Input: part model. Units: mm. Frame: model coordinates. Face numbers are marked on the shaded views. Round coordinates to 2 decimals unless told otherwise and drop trailing zeros. Loops run counter-clockwise (first coordinate to the right, second up) from the corner with the lowest first, then second, coordinate; pieces in that order, holes last.
1) Section B-B, the plane z = 0. Return loops of the section in (x, y).
2) Section C-C, the plane y = -35. Return loops of the section in (x, z).
3) First-contact query: pin 1 (1.5 mm diameter, centred on x = -31.5, y = -41.5, fed in from -Z). Flat tip, straight axial feed; report the tip coordinate or a pass-through.
4) Section A-A, the plane x = 0. Return loops of the section in (y, z), and give its area (3 significant figures).
5) Ray query, line 1 along Z through (x, y) = (0, -13); line 2 along Z through (x, y) = (3.5, -42.5); line 3 along X through (y, z) = (-47.5, -14). Return the intervals inside material, ascending.
6) Section D-D, the plane x = -30. Return loops of the section in (y, z), and give its area (3 significant figures).
7) Draft query along X for the marked faces 1, 2 and 3. Return one class per face: pulls with the +X half, pulls with the -X half, needs draft (parallel to the pull), parting line crosses it, or undercut.
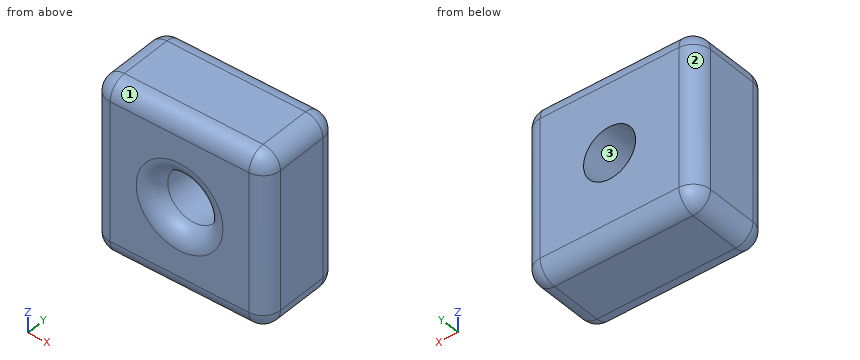
from build123d import *

# Parameters (mm, degrees)
F0_W     = 100
F0_H     = 100
F0_R     = 15
F1_DEPTH = 50
F2_R     = 10
F3_DEPTH = 50
F6_R     = 10


# Not quite as in the source:
# - the program builds the solid bodies; features that only make, move or delete a surface that nothing else refers to are left out


with BuildPart() as f1:
    # F0 (on Front) → F1 (new body, symmetric)
    with BuildSketch(Plane.XZ):
        Rectangle(F0_W, F0_H)
        Circle(F0_R, mode=Mode.SUBTRACT)
    extrude(amount=F1_DEPTH, both=True)

    # F2
    f2_edges = [f1.edges().sort_by_distance(p)[0] for p in [
        (50, 50, 0),
        (50, 0, 50),
        (50, -50, 0),
        (50, 0, -50),
        (0, -50, 50),
        (-50, -50, 0),
        (0, -50, -50),
        (-15, -50, 0),
        (0, 50, 50),
        (-50, 0, 50),
        (-50, 50, 0),
        (-50, 0, -50),
    ]]
    fillet(f2_edges, radius=F2_R)

    # F0 (on Front) → F3 (cut)
    with BuildSketch(Plane.XZ):
        Rectangle(F0_W, F0_H)
        Circle(F0_R, mode=Mode.SUBTRACT)
    extrude(amount=-F3_DEPTH, mode=Mode.SUBTRACT)

    # F6
    f6_edges = [f1.edges().sort_by_distance(p)[0] for p in [
        (-47.071068, 0, -47.071068),
        (-40, -20, -50),
        (-47.071068, -40, -47.071068),
        (-50, -20, -40),
        (-47.071068, 0, 47.071068),
        (-40, -20, 50),
        (-47.071068, -40, 47.071068),
        (-50, -20, 40),
        (-47.071068, -47.071068, 40),
        (-50, -40, 0),
        (-40, -50, 0),
        (-47.071068, -47.071068, -40),
        (-50, 0, 0),
        (47.071068, -40, -47.071068),
        (50, -20, -40),
        (47.071068, 0, -47.071068),
        (40, -20, -50),
        (50, -40, 0),
        (50, -20, 40),
        (50, 0, 0),
        (40, -50, 0),
        (0, -50, -40),
        (0, -50, 40),
        (-25, -50, 0),
        (0, 0, 50),
        (47.071068, 0, 47.071068),
        (0, 0, -50),
    ]]
    fillet(f6_edges, radius=F6_R)


solid = f1.part
Final values:
1. outline: (-50, -40) arc R10 ccw to (-40, -50) - (-25, -50) arc R10 ccw to (-15, -40) - (-15, 0) - (-40, 0) arc R10 ccw to (-50, -10) - close; (15, -40) arc R10 ccw to (25, -50) - (40, -50) arc R10 ccw to (50, -40) - (50, -10) arc R10 ccw to (40, 0) - (15, 0) - close
2. outline: (-50, -40) arc R10 ccw to (-40, -50) - (40, -50) arc R10 ccw to (50, -40) - (50, 40) arc R10 ccw to (40, 50) - (-40, 50) arc R10 ccw to (-50, 40) - close; hole circle Ø30 at (0, 0)
3. pin 1: stops at z = -49.97
4. outline: (-50, -40) arc R10 ccw to (-40, -50) - (-10, -50) arc R10 ccw to (0, -40) - (0, -15) - (-40, -15) arc R10 ccw to (-50, -25) - close; (-50, 25) arc R10 ccw to (-40, 15) - (0, 15) - (0, 40) arc R10 ccw to (-10, 50) - (-40, 50) arc R10 ccw to (-50, 40) - close
4. area: 3,370 mm2
5. line 1: z = -50 to -15, 15 to 50
5. line 2: z = -49.68 to -14.91, 14.91 to 49.68
5. line 3: x = -46.61 to -11.92, 11.92 to 46.61
6. outline: (-50, -40) arc R10 ccw to (-40, -50) - (-10, -50) arc R10 ccw to (0, -40) - (0, 40) arc R10 ccw to (-10, 50) - (-40, 50) arc R10 ccw to (-50, 40) - close
6. area: 4,910 mm2
7. face 1: needs draft
7. face 2: pulls with the -X half
7. face 3: undercut
